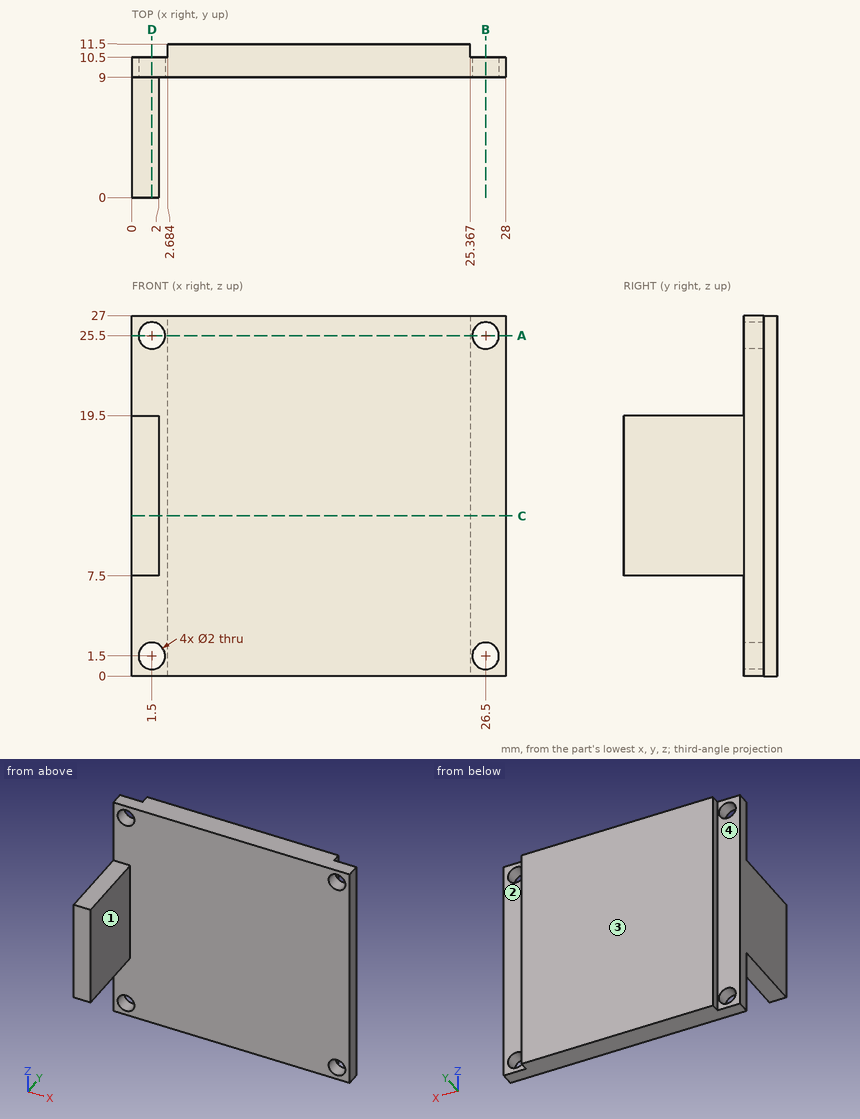
Study the drawing (mm; zero at the part's minimum x, y, z) and answer. A direction names the side the tool comes from. Coordinates: 2 decimals unless noted, no trailing zeros. Write each loop counter-clockwise with the first axis right and the second up, starting at its lowest first coordinate (ties: lowest second). Pieces come first, ordered by that corner, then holes. Notation, with made-up numbers: (27.5, 66) - (31.5, 66) arc R17 ccw to (31.5, 86) - close; hole circle Ø9 at (-19.75, -1). An arc over 180 degrees is marked (long way). Put each result on its own line as item: value.
1. The part is cut by section C-C on z = 12. Give the vertices of the cut face in (x, y).
Answer sheet:
outline: (0, 0) - (2, 0) - (2, 9) - (28, 9) - (28, 10.5) - (25.37, 10.5) - (25.37, 11.5) - (2.68, 11.5) - (2.68, 10.5) - (0, 10.5) - close
2. Find the intervals of material crossed by line 1 along Z through (x, y) = (26.5, 10.2); line 2 along X through (y, z) = (9.75, 25.5); line 3 along Y through (x, z) = (10.5, 9.5), in increasing order. Write a range as from..to.
Answer sheet:
line 1: z = 0..0.5, 2.5..24.5, 26.5..27
line 2: x = 0..0.5, 2.5..25.5, 27.5..28
line 3: y = 9..11.5
3. The part is cut by section B-B on x = 26.5. Give the vertices of the cut face in (y, z), plus the area to 3 significant figures.
Answer sheet:
outline: (9, 0) - (10.5, 0) - (10.5, 0.5) - (9, 0.5) - close; (9, 2.5) - (10.5, 2.5) - (10.5, 24.5) - (9, 24.5) - close; (9, 26.5) - (10.5, 26.5) - (10.5, 27) - (9, 27) - close
area: 34.5 mm^2
4. The part is cut by section A-A on z = 25.5. Give the vertices of the cut face in (x, y).
Answer sheet:
outline: (0, 9) - (0.5, 9) - (0.5, 10.5) - (0, 10.5) - close; (2.5, 9) - (25.5, 9) - (25.5, 10.5) - (25.37, 10.5) - (25.37, 11.5) - (2.68, 11.5) - (2.68, 10.5) - (2.5, 10.5) - close; (27.5, 9) - (28, 9) - (28, 10.5) - (27.5, 10.5) - close
5. Flat-ended cylindrical pins translate along their axes: pin 1 Ø1.3 at (x, z) = (1.5, 17.5) entering from +Y; pin 2 Ø5 at (x, z) = (22.5, 23) entering from -Y; pin 3 Ø6 at (y, z) = (2.5, 8.5) entering from +X. Find the tip coordinate at first contact, or state that the pin passes through.
Answer sheet:
pin 1: stops at y = 10.5
pin 2: stops at y = 9
pin 3: stops at x = 2
6. A tool of negligible diameter and unlimited length cuts with its end or side. For the marked faces 1, 2, 3 and 4, from which of +Z, -Z, +X, -X, +Y, -Y can it reach the whole face along a straight path? Write none if from no direction.
Answer sheet:
face 1: +Z, -Z, +X, -Y
face 2: +Z, -Z, +X, +Y
face 3: +Z, -Z, +X, -X, +Y
face 4: +Z, -Z, -X, +Y
7. The part is cut by section D-D on x = 1.5. Give the vertices of the cut face in (y, z), plus the area to 4 significant figures.
Answer sheet:
outline: (0, 7.5) - (9, 7.5) - (9, 2.5) - (10.5, 2.5) - (10.5, 24.5) - (9, 24.5) - (9, 19.5) - (0, 19.5) - close; (9, 0) - (10.5, 0) - (10.5, 0.5) - (9, 0.5) - close; (9, 26.5) - (10.5, 26.5) - (10.5, 27) - (9, 27) - close
area: 142.5 mm^2
